from build123d import *

# Parameters (mm, degrees)
SKETCH1_R           = 90
SKETCH1_R_2         = 80
BOSS_EXTRUDE1_DEPTH = 10
SKETCH2_R           = 2.5
SKETCH3_W           = 200
SKETCH3_H           = 15
BOSS_EXTRUDE2_DEPTH = 10
SKETCH5_W           = 60
SKETCH5_H           = 95
SKETCH5_R           = 1.5
BOSS_EXTRUDE3_DEPTH = 10
SKETCH7_W           = 44.3
SKETCH7_H           = 44.3
SKETCH7_W_2         = 42.3
SKETCH7_H_2         = 42.3
BOSS_EXTRUDE4_DEPTH = 5
SKETCH8_W           = 95
SKETCH8_H           = 30
BOSS_EXTRUDE5_DEPTH = 35
BOSS_EXTRUDE7_DEPTH = 5
SKETCH10_R          = 5
CUT_EXTRUDE1_DEPTH  = 212.187120819


with BuildPart() as part:
    # Sketch1 → Boss-Extrude1 (new body)
    with BuildSketch(Plane(origin=(0, 0, 0), x_dir=(1, 0, 0), z_dir=(0, 1, 0))):
        with Locations(Location((0, 0, 0), (0, 0, 270))):
            Circle(SKETCH1_R)
        with Locations(Location((0, 0, 0), (0, 0, 270))):
            Circle(SKETCH1_R_2, mode=Mode.SUBTRACT)
    extrude(amount=BOSS_EXTRUDE1_DEPTH)

    # Sketch2 → Cut-Revolve1 (revolve, cut)
    with BuildSketch(Plane.XY, mode=Mode.PRIVATE) as cut_revolve1_sk:
        with Locations((-85, 0)):
            Circle(SKETCH2_R)
    revolve(cut_revolve1_sk.sketch.rotate(Axis((0, 0, 0), (0, 1, 0)), 270), axis=Axis((0, 0, 0), (0, 1, 0)), mode=Mode.SUBTRACT)

    # Sketch3 → Boss-Extrude2 (add)
    with BuildSketch(Plane(origin=(0, 10, 0), x_dir=(1, 0, 0), z_dir=(0, 1, 0))):
        with Locations((0, -40)):
            Rectangle(SKETCH3_W, SKETCH3_H)
        with Locations((0, 40)):
            Rectangle(SKETCH3_W, SKETCH3_H)
    extrude(amount=BOSS_EXTRUDE2_DEPTH)

    # Sketch5 → Boss-Extrude3 (add)
    with BuildSketch(Plane.XZ.offset(-10)):
        with Locations((-130, 0)):
            Rectangle(SKETCH5_W, SKETCH5_H)
        with Locations(Location((-145.5, -15.5, 0), (0, 0, 270))):
            Circle(SKETCH5_R, mode=Mode.SUBTRACT)
        with Locations(Location((-114.5, -15.5, 0), (0, 0, 270))):
            Circle(SKETCH5_R, mode=Mode.SUBTRACT)
        with Locations(Location((-114.5, 15.5, 0), (0, 0, 270))):
            Circle(SKETCH5_R, mode=Mode.SUBTRACT)
        with Locations(Location((-145.5, 15.5, 0), (0, 0, 270))):
            Circle(SKETCH5_R, mode=Mode.SUBTRACT)
    extrude(amount=-BOSS_EXTRUDE3_DEPTH)

    # Sketch7 → Boss-Extrude4 (add)
    with BuildSketch(Plane.XZ.offset(-10)):
        with Locations((-130, 0)):
            Rectangle(SKETCH7_W, SKETCH7_H)
        with Locations((-130, 0)):
            Rectangle(SKETCH7_W_2, SKETCH7_H_2, mode=Mode.SUBTRACT)
    extrude(amount=BOSS_EXTRUDE4_DEPTH)

    # Sketch8 → Boss-Extrude5 (add, symmetric)
    with BuildSketch(Plane(origin=(0, 0, 0), x_dir=(0, 0, -1), z_dir=(1, 0, 0))):
        with Locations((0, 35)):
            Rectangle(SKETCH8_W, SKETCH8_H)
    extrude(amount=BOSS_EXTRUDE5_DEPTH, both=True)

    # Sketch9 → Boss-Extrude7 (add)
    with BuildSketch(Plane.ZY.offset(35)):
        Polygon((-47.5, 50), (0, 130), (47.5, 50), (47.5, 20), (-47.5, 20), align=None)
    boss_extrude7 = extrude(amount=BOSS_EXTRUDE7_DEPTH)

    # Mirror1: Boss-Extrude7 across plane
    add(boss_extrude7.mirror(Plane(origin=(0, 0, 0), x_dir=(0, 0, 1), z_dir=(1, 0, 0))))

    # Sketch10 → Cut-Extrude1 (cut, through all)
    with BuildSketch(Plane.ZY.offset(40)):
        with Locations(Location((0, 95, 0), (0, 0, 180))):
            Circle(SKETCH10_R)
    extrude(amount=-CUT_EXTRUDE1_DEPTH, mode=Mode.SUBTRACT)


solid = part.part
Geometry check sheet. Reference: the model listing, model coordinates, mm. A direction names the side the tool comes from. Round coordinates to 2 decimals unless told otherwise and drop trailing zeros. Order: outer loops, then holes, each group sorted by start corner. A loop starts at its lowest first (then second) coordinate and runs counter-clockwise, first axis right, second up. Notation, with made-up numbers: M 85.25,9 L 98.25,9 A5 ccw 98.25,18 Z; hole C 87,40.25 d6. An arc over 180 degrees is marked long. Answer in a Markdown table with one row per item.
(1) Sectioned sample at A-A, the plane x = 0. Record the cut outline in (y, z).
Responses:
| item | result |
|---|---|
| outline | M 0,-90 L 10,-90 L 10,-80 L 0,-80 L 0,-82.5 A2.5 cw 0,-87.5 Z; M 0,80 L 10,80 L 10,90 L 0,90 L 0,87.5 A2.5 cw 0,82.5 Z; M 10,-47.5 L 50,-47.5 L 50,47.5 L 10,47.5 L 10,32.5 L 20,32.5 L 20,-32.5 L 10,-32.5 Z |
(2) Go/stop test with flat-tipped pins: P1, Ø5, axis at y = 17, z = -3, coming from the +X side; P2, Ø13, axis at y = 95, z = 0, coming from the -X side; P3, Ø4, axis at x = 35.5, y = 97, coming from the +Z side; P4, Ø12, axis at x = -58, y = 26.5, coming from the +Z side. Record where each tip stops, or that it passes through.
Responses:
| item | result |
|---|---|
| P1 | stops at x = -100 |
| P2 | stops at x = -40 |
| P3 | stops at z = 20.78 |
| P4 | passes through |
(3) Sectioned sample at B-B, the plane y = 104.5. Record the cut outline in (x, z), and give its area (3 significant figures).
Responses:
| item | result |
|---|---|
| outline | M -40,-15.14 L -35,-15.14 L -35,15.14 L -40,15.14 Z; M 35,-15.14 L 40,-15.14 L 40,15.14 L 35,15.14 Z |
| area | 303 mm² |
(4) Sectioned sample at C-C, the plane x = -137. Record the cut outline in (y, z).
Responses:
| item | result |
|---|---|
| outline | M 5,-22.15 L 10,-22.15 L 10,-47.5 L 20,-47.5 L 20,47.5 L 10,47.5 L 10,22.15 L 5,22.15 L 5,21.15 L 10,21.15 L 10,-21.15 L 5,-21.15 Z |
(5) Tool access check on faces 1 (the face through (91, 10, -40)), 2 (the face through (-35, 73, 1)), 3 (the face through (84, 10, 0)). Record the directions out of +Z, -Z, +X, -X, +Y, -Y that give a thin tool (end or side, any length) a straight path to the whole face; none if there is none.
Responses:
| item | result |
|---|---|
| face 1 | -Z, +X, -Y |
| face 2 | +Z, -Z, +Y |
| face 3 | +X, +Y |
(6) Sectioned sample at D-D, the plane z = 8. State how many separate pieces and enclosed holes the cut face has, and give its area (3 significant figures).
Responses:
| item | result |
|---|---|
| separate pieces | 4 |
| enclosed holes | 0 |
| area | 3,860 mm² |
(7) Scan lines: probe 1 along Z at (x, y) = (0, 4); probe 2 along Z at (x, y) = (-114, 13); probe 3 along Y at (x, z) = (-102.5, -25.5). Record each from-to range of solid material in increasing order. Write a range as from..to.
Responses:
| item | result |
|---|---|
| probe 1 | z = -90..-80, 80..90 |
| probe 2 | z = -47.5..-16.91, -14.09..14.09, 16.91..47.5 |
| probe 3 | y = 10..20 |
(8) Draft check along Z on faces 4 (the face through (37.465, 90.56, 23.418)), 5 (the face through (-1, 15, 32.5)), 6 (the face through (-40, 64, 1)). Enter one of: released by +Z, released by -Z, zero draft, split by the parting line, or undercut.
Responses:
| item | result |
|---|---|
| face 4 | released by +Z |
| face 5 | undercut |
| face 6 | zero draft |
